from build123d import *

# Parameters (mm, degrees)
F0_R     = 5
F1_DEPTH = 9.5
F2_SIZE  = 1.5
F4_R     = 6
F5_DEPTH = 1
F3_W     = 5.5
F3_H     = 3.5
F6_DEPTH = 9


with BuildPart() as f1:
    # F0 (on Top) → F1 (new body)
    with BuildSketch(Plane.XY):
        Circle(F0_R)
    extrude(amount=F1_DEPTH)

    # F2
    f2_edges = [f1.edges().sort_by_distance(p)[0] for p in [
        (-5, 0, 9.5),
    ]]
    chamfer(f2_edges, length=F2_SIZE)

    # F4 (on face) → F5 (join)
    with BuildSketch(Plane.XY):
        Circle(F4_R)
    extrude(amount=-F5_DEPTH)

    # F3 (on face) → F6 (cut)
    with BuildSketch(Plane.XY.offset(9.5)):
        Rectangle(F3_W, F3_H)
    extrude(amount=-F6_DEPTH, mode=Mode.SUBTRACT)


solid = f1.part
Read the model definition and answer for the solid it produces. Units are mm, in the model's axes. A direction names the side the tool comes from. Coordinates: 2 decimals unless noted, no trailing zeros. Write each loop counter-clockwise with the first axis right and the second up, starting at its lowest first coordinate (ties: lowest second). Pieces come first, ordered by that corner, then holes. Notation, with made-up numbers: (26, 49) - (74, 49) arc R23 ccw to (74, 58) - close; hole circle Ø3 at (35, 12). An arc over 180 degrees is marked (long way). One line per question, with ' | ' between items.
Q1. Determine the mould class of faces 1 (the cylindrical face through (-5.994, 0.264, -0.493)), 2 (the flat face through (0, 1.75, 5)), 3 (the flat face through (-2.75, 0, 5)), 4 (the flat face through (0, -2, 9.5)) for opening direction Y: +Y half, -Y half, draft (parallel to the pull), parting line (faces both ways), or undercut.
Result set:
face 1: parting line | face 2: undercut | face 3: undercut | face 4: draft
Q2. Each of these flat-tipped pins is pushed along its axis until it touches: P1, Ø1, axis at x = -3, z = 7.5, coming from the +Y side; P2, Ø1.8, axis at y = 0, z = 7, coming from the +X side; P3, Ø2, axis at x = -1.5, z = 7.5, coming from the +Y side. Where does it stop, or does it pass through?
Result set:
P1: y = 4.33 | P2: x = 5 | P3: y = 4.97
Q3. Find section C-C, the plane y = 0. Write down the section's boundary in (x, z).
Result set:
outline: (-6, -1) - (6, -1) - (6, 0) - (5, 0) - (5, 8) - (3.5, 9.5) - (2.75, 9.5) - (2.75, 0.5) - (-2.75, 0.5) - (-2.75, 9.5) - (-3.5, 9.5) - (-5, 8) - (-5, 0) - (-6, 0) - close
Q4. Find section D-D, the plane z = 9.25. Write down the section's boundary in (x, y).
Result set:
outline: circle Ø7.5 at (0, 0); hole (-2.75, -1.75) - (2.75, -1.75) - (2.75, 1.75) - (-2.75, 1.75) - close
Q5. Find section A-A, the plane z = 6.25. Write down the section's boundary in (x, y), plus the area to 3 significant figures.
Result set:
outline: circle Ø10 at (0, 0); hole (-2.75, -1.75) - (2.75, -1.75) - (2.75, 1.75) - (-2.75, 1.75) - close | area: 59.3 mm^2
Q6. For faces 5 (the flat face through (2.75, 0, 5)), 6 (the flat face through (0, 0, -1)), determine the directions among +Z, -Z, +X, -X, +Y, -Y from which every point of the face is accessible in a straight line to the end or side of a thin tool.
Result set:
face 5: +Z | face 6: -Z, +X, -X, +Y, -Y
Q7. Find section B-B, the plane x = 0. Write down the section's boundary in (y, z).
Result set:
outline: (-6, -1) - (6, -1) - (6, 0) - (5, 0) - (5, 8) - (3.5, 9.5) - (1.75, 9.5) - (1.75, 0.5) - (-1.75, 0.5) - (-1.75, 9.5) - (-3.5, 9.5) - (-5, 8) - (-5, 0) - (-6, 0) - close
Q8. Consider L1, parallel to X at y = 0.5, z = 1.5; L2, parallel to Y at x = -2.25, z = 4.5; L3, parallel to X at y = -0.75, z = 2.25. Determine where each line is inside the solid, lowest interval first. Write a range as [from, to].
Result set:
L1: [-4.97, -2.75], [2.75, 4.97] | L2: [-4.47, -1.75], [1.75, 4.47] | L3: [-4.94, -2.75], [2.75, 4.94]
